```python
from build123d import *

# Parameters (mm, degrees)
F1_DEPTH = 405
F2_T     = -1.5
F3_DEPTH = 5
F5_DEPTH = 3
F6_DEPTH = 2
F7_W     = 10
F7_H     = 5
F8_DEPTH = 15
F9_R     = 4.99999
F11_D    = 5


# Not quite as in the source:
# - a fillet or chamfer is up to 0.001 mm smaller than in the source, because OpenCascade refuses the exact size


with BuildPart() as f1:
    # F0 (on Front) → F1 (new body)
    with BuildSketch(Plane.XZ):
        with BuildLine():
            Line((-210, -105), (210, -105))
            Line((210, -105), (210, 105))
            ThreePointArc((210, 105), (0, 135), (-210, 105))
            Line((-210, 105), (-210, -105))
        make_face()
    extrude(amount=-F1_DEPTH)

    # F2
    f2_openings = [f1.faces().sort_by_distance(p)[0] for p in [
        (0, 0, 10.213522),
    ]]
    offset(amount=F2_T, openings=f2_openings)

    # F0 (on Front) → F3 (join)
    with BuildSketch(Plane.XZ):
        with BuildLine():
            ThreePointArc((245, 141.3068160476), (0, 180), (-245, 141.3068160476))
            Line((-245, 141.3068160476), (-245, -140))
            Line((-245, -140), (245, -140))
            Line((245, -140), (245, 141.3068160476))
        make_face()
        with BuildLine():
            Line((210, 105), (210, -105))
            Line((210, -105), (-210, -105))
            Line((-210, -105), (-210, 105))
            ThreePointArc((-210, 105), (0, 135), (210, 105))
        make_face(mode=Mode.SUBTRACT)
    extrude(amount=-F3_DEPTH)

    # F4 (on face) → F5 (join)
    with BuildSketch(Plane.XZ):
        with BuildLine():
            Line((245, -140), (245, 141.3068160476))
            ThreePointArc((245, 141.3068160476), (0, 180), (-245, 141.3068160476))
            Line((-245, 141.3068160476), (-245, -140))
            Line((-245, -140), (245, -140))
        make_face()
        with BuildLine():
            Line((-242, -137), (-242, 139.1220060441))
            ThreePointArc((-242, 139.1220060441), (0, 177), (242, 139.1220060441))
            Line((242, 139.1220060441), (242, -137))
            Line((242, -137), (-242, -137))
        make_face(mode=Mode.SUBTRACT)
    extrude(amount=F5_DEPTH)

    # F4 (on face) → F6 (join)
    with BuildSketch(Plane.XZ):
        with BuildLine():
            ThreePointArc((213, 117.6663633606), (0, 148), (-213, 117.6663633606))
            Line((-213, 117.6663633606), (-213, -108))
            Line((-213, -108), (213, -108))
            Line((213, -108), (213, 117.6663633606))
        make_face()
        with BuildLine():
            ThreePointArc((-210, 115.410843293), (0, 145), (210, 115.410843293))
            Line((210, 115.410843293), (210, 105))
            Line((210, 105), (210, -105))
            Line((210, -105), (-210, -105))
            Line((-210, -105), (-210, 105))
            Line((-210, 105), (-210, 115.410843293))
        make_face(mode=Mode.SUBTRACT)
    extrude(amount=F6_DEPTH)

    # F7 (on face) → F8 (join)
    with BuildSketch(Plane.XZ):
        with Locations((240, 112.5)):
            Rectangle(F7_W, F7_H)
        with Locations((240, -112.5)):
            Rectangle(F7_W, F7_H)
    extrude(amount=F8_DEPTH)

    # F9 (radius 5 in the source; OpenCascade refuses exactly that, so slightly less here)
    f9_edges = [f1.edges().sort_by_distance(p)[0] for p in [
        (245, -15, 112.5),
        (235, -15, 112.5),
        (245, -15, -112.5),
        (235, -15, -112.5),
    ]]
    fillet(f9_edges, radius=F9_R)

    # F11 (through all)
    with Locations(Plane.XY.offset(115)):
        with Locations((240, -10)):
            Hole(F11_D / 2)


solid = f1.part
```
Check sheet for the modelled part. Datum: model origin and axes. Units: mm. A direction names the side the tool comes from. Give positions to 0.01 mm unless a question says otherwise; leave off trailing zeros. Order: outer loops, then holes, each group sorted by start corner. A loop starts at its lowest first (then second) coordinate and runs counter-clockwise, first axis right, second up. Notation, with made-up numbers: M 49,16 L 77,16 A21 ccw 77,40 Z; hole C 57.5,80 d10. An arc over 180 degrees is marked long. Answer in a Markdown table with one row per item.
1) Cross-section at B-B, the plane z = 89. Enter the section's corners in (x, y), plus the area to 3 significant figures.
Filled sheet:
| item | result |
|---|---|
| outline | M -245,-3 L -242,-3 L -242,0 L -213,0 L -213,-2 L -210,-2 L -210,0 L -208.5,0 L -208.5,403.5 L 208.5,403.5 L 208.5,0 L 210,0 L 210,-2 L 213,-2 L 213,0 L 242,0 L 242,-3 L 245,-3 L 245,5 L 210,5 L 210,405 L -210,405 L -210,5 L -245,5 Z |
| area | 2,220 mm2 |
2) Gauge pin test, flat ends, axial feed: P1, Ø1, axis at x = -88, y = 271, coming from the +Z side; P2, Ø8, axis at x = 240, y = -10, coming from the +Z side; P3, Ø1.5, axis at y = -6, z = -113, coming from the -X side. Record the tip position at first contact, or that the pin passes through.
Filled sheet:
| item | result |
|---|---|
| P1 | stops at z = 129.88 |
| P2 | stops at z = 115 |
| P3 | stops at x = 235 |
3) Access from +Z, -Z, +X, -X, +Y, -Y to the whole of each face (thin tool, end or side, straight path). Record for faces 1 (the cylindrical face through (2.958, 198.926, 133.494)), 2 (the flat face through (245, 1, -1)), 3 (the flat face through (-210, 202, 1)), 4 (the flat face through (-3, 405, 17)), 5 (the flat face through (-3, 202, -105)).
Filled sheet:
| item | result |
|---|---|
| face 1 | -Y |
| face 2 | +Z, -Z, +X, +Y, -Y |
| face 3 | +Z, -Z, -X, +Y |
| face 4 | +Z, -Z, +X, -X, +Y |
| face 5 | -Z, +X, -X, +Y |
4) Cross-section at C-C, the plane x = 180.5. Enter the section's corners in (y, z), plus the area to 3 significant figures.
Filled sheet:
| item | result |
|---|---|
| outline | M -3,-140 L 5,-140 L 5,-105 L 405,-105 L 405,112.96 L 5,112.96 L 5,159.24 L -3,159.24 L -3,156.16 L 0,156.16 L 0,126.34 L -2,126.34 L -2,123.25 L 0,123.25 L 0,111.41 L 403.5,111.41 L 403.5,-103.5 L 0,-103.5 L 0,-105 L -2,-105 L -2,-108 L 0,-108 L 0,-137 L -3,-137 Z |
| area | 1,990 mm2 |
5) Thickness scan on L1, parallel to X at y = 36.5, z = 35.5; L2, parallel to Z at x = 11, y = 356.5; L3, parallel to Z at x = -68, y = 226.5. Record the ranges inside material, lowest first. Write a range as [from, to].
Filled sheet:
| item | result |
|---|---|
| L1 | x = [-210, -208.5], [208.5, 210] |
| L2 | z = [-105, -103.5], [133.42, 134.92] |
| L3 | z = [-105, -103.5], [130.4, 131.91] |
6) Release check for a two-part mould opening along Z. For faces 6 (the cylindrical face through (3.022, -0.986, 147.994)), 7 (the flat face through (210, 202, -1)), 8 (the cylindrical face through (2.98, 202.2, 134.994)) record: +Z half, -Z half, draft (parallel to the pull), parting line (faces both ways), or undercut.
Filled sheet:
| item | result |
|---|---|
| face 6 | undercut |
| face 7 | draft |
| face 8 | +Z half |
7) Cross-section at A-A, the plane y = 244. Enter the section's corners in (x, z).
Filled sheet:
| item | result |
|---|---|
| outline | M -210,-105 L 210,-105 L 210,105 A750 ccw -210,105 Z; hole M -208.5,-103.5 L 208.5,-103.5 L 208.5,103.87 A748.5 ccw -208.5,103.87 Z |
